from build123d import *

# Parameters (mm, degrees)
F0_R     = 8.5
F1_DEPTH = 16.5
F2_W     = 1.2
F2_H     = 1.2
F3_DEPTH = 5
F4_DEPTH = 9
F5_SIZE  = 0.15


with BuildPart() as f1:
    # F0 (on Top) → F1 (new body)
    with BuildSketch(Plane.XY):
        Circle(F0_R)
    extrude(amount=F1_DEPTH)

    # F2 (on face) → F3 (join)
    with BuildSketch(Plane(origin=(0, 0, 0), x_dir=(1, 0, 0), z_dir=(0, 0, -1))):
        with Locations((-3.75, 0)):
            Rectangle(F2_W, F2_H)
    extrude(amount=F3_DEPTH)

    # F2 (on face) → F4 (join)
    with BuildSketch(Plane(origin=(0, 0, 0), x_dir=(1, 0, 0), z_dir=(0, 0, -1))):
        with Locations((3.75, 0)):
            Rectangle(F2_W, F2_H)
    extrude(amount=F4_DEPTH)

    # F5
    f5_edges = [f1.edges().sort_by_distance(p)[0] for p in [
        (-3.75, -0.6, -5),
        (-4.35, 0, -5),
        (-3.75, 0.6, -5),
        (-3.15, 0, -5),
        (3.15, 0, -9),
        (3.75, -0.6, -9),
        (4.35, 0, -9),
        (3.75, 0.6, -9),
    ]]
    chamfer(f5_edges, length=F5_SIZE)


solid = f1.part
Can you work these out from the model? Positions are in its coordinate system, mm. A direction names the side the tool comes from. Round coordinates to 2 decimals unless told otherwise and drop trailing zeros. Write each loop counter-clockwise with the first axis right and the second up, starting at its lowest first coordinate (ties: lowest second). Pieces come first, ordered by that corner, then holes. Notation, with made-up numbers: (-24, 7.5) -> (22, 7.5) arc R32 ccw to (22, 41.5) -> close; hole circle Ø8 at (79.25, -12.5). An arc over 180 degrees is marked (long way). Use one line per item in the form item = value. Start each with the question number.
Q1. Imagine slicing it at D-D (x = -2.5). Please give me the cut outline in (y, z).
Q2. I'm going to push flat-ended pins straight in: P1, Ø5, axis at x = -0.5, y = 6, coming from the -Z side; P2, Ø0.6, axis at x = -4, z = -3, coming from the -Y side; P3, Ø4, axis at y = 3, z = 1.5, coming from the +X side; P4, Ø8, axis at y = -0.5, z = 9.5, coming from the +X side. Where does each tip first touch, or does it pass through?
Q3. We'd pull the mould along X, two halves only. Please class faces 1 (the face through (-4, -0.6, -2)), 2 (the face through (3.15, 0, -4)), 3 (the face through (4.57, 7.167, 8.134)), 4 (the face through (-3.15, 0, -2)): +X half, -X half, draft (parallel to the pull), parting line (faces both ways), or undercut.
Q4. If I drill on probe 1 along Z at (x, y) = (-6.75, -1.5); probe 2 along Y at (x, z) = (-3.75, -2); probe 3 along X at (y, z) = (-0.25, 5), over which ranges is the centre line in solid material (lowest first)? Write a range as [from, to].
Q5. Imagine slicing it at B-B (x = 0). Please give me the cut outline in (y, z).
Q6. Imagine slicing it at A-A (y = 0). Please give me the cut outline in (x, z).
Q7. Imagine slicing it at C-C (z = 2.25). Please give me the cut outline in (x, y), then the cut area to 3 significant figures.
Q8. Which directions (+Z, -Z, +X, -X, +Y, -Y) give clear straight access to the entire face, cutting with the end or side of a thin tool? Please do faces 5 (the face through (4.35, 0, -4)), 6 (the face through (4, 0.6, -4)), 7 (the face through (0, 0, 16.5)), 8 (the face through (-4, 0, -5)), 9 (the face through (4, -0.6, -4)).
Worked out:
q1.outline = (-8.12, 0) -> (8.12, 0) -> (8.12, 16.5) -> (-8.12, 16.5) -> close
q2.P1 = 0
q2.P2 = -0.6
q2.P3 = 8.44
q2.P4 = 8.5
q3.face_1 = draft
q3.face_2 = undercut
q3.face_3 = parting line
q3.face_4 = undercut
q4.probe_1 = [0, 16.5]
q4.probe_2 = [-0.6, 0.6]
q4.probe_3 = [-8.5, 8.5]
q5.outline = (-8.5, 0) -> (8.5, 0) -> (8.5, 16.5) -> (-8.5, 16.5) -> close
q6.outline = (-8.5, 0) -> (-4.35, 0) -> (-4.35, -4.85) -> (-4.2, -5) -> (-3.3, -5) -> (-3.15, -4.85) -> (-3.15, 0) -> (3.15, 0) -> (3.15, -8.85) -> (3.3, -9) -> (4.2, -9) -> (4.35, -8.85) -> (4.35, 0) -> (8.5, 0) -> (8.5, 16.5) -> (-8.5, 16.5) -> close
q7.outline = circle Ø17 at (0, 0)
q7.area = 227 mm^2
q8.face_5 = -Z, +X, +Y, -Y
q8.face_6 = -Z, +X, -X, +Y
q8.face_7 = +Z, +X, -X, +Y, -Y
q8.face_8 = -Z, -X, +Y, -Y
q8.face_9 = -Z, +X, -X, -Y
